```python
from build123d import *

# Parameters (mm, degrees)
F0_W     = 660.4
F0_H     = 571.5
F0_R     = 6.746875
F1_DEPTH = 2.3876
F3_DEPTH = 2.3886
F4_W     = 381
F4_H     = 292.1
F5_DEPTH = 2.3886


with BuildPart() as f1:
    # F0 (on Top) → F1 (new body)
    with BuildSketch(Plane.XY):
        Rectangle(F0_W, F0_H)
        with Locations((-233.3625, -233.3625)):
            Circle(F0_R, mode=Mode.SUBTRACT)
        with Locations((-252.96602, -198.4248)):
            Circle(F0_R, mode=Mode.SUBTRACT)
        with Locations((233.3625, -233.3625)):
            Circle(F0_R, mode=Mode.SUBTRACT)
        with Locations((252.96602, -198.4248)):
            Circle(F0_R, mode=Mode.SUBTRACT)
        with Locations((-233.3625, 233.3625)):
            Circle(F0_R, mode=Mode.SUBTRACT)
        with Locations((0, 239.7252)):
            Circle(F0_R, mode=Mode.SUBTRACT)
        with Locations((233.3625, 233.3625)):
            Circle(F0_R, mode=Mode.SUBTRACT)
    extrude(amount=-F1_DEPTH)

    # F2 (on Top) → F3 (cut, through all)
    with BuildSketch(Plane.XY):
        Polygon((22.225, 285.75), (-22.225, 285.75), (0, 263.525), align=None)
        Polygon((-22.225, -285.75), (22.225, -285.75), (0, -263.525), align=None)
    extrude(amount=-F3_DEPTH, mode=Mode.SUBTRACT)

    # F4 (on Top) → F5 (cut, through all)
    with BuildSketch(Plane.XY):
        Rectangle(F4_W, F4_H)
    extrude(amount=-F5_DEPTH, mode=Mode.SUBTRACT)


solid = f1.part
```
Read the model definition and answer for the solid it produces. Units are mm, in the model's axes. A direction names the side the tool comes from. Round coordinates to 2 decimals unless told otherwise and drop trailing zeros. Write each loop counter-clockwise with the first axis right and the second up, starting at its lowest first coordinate (ties: lowest second). Pieces come first, ordered by that corner, then holes. Notation, with made-up numbers: M 38,-13.5 L 69,-13.5 A27 ccw 69,5.5 Z; hole C 63.5,63 d3. An arc over 180 degrees is marked long. One line per item, written item: value.
Q1. Which of the six approach directions +Z, -Z, +X, -X, +Y, -Y give full straight-line access (tool end or side, diameter ignored) to faces 3 (the flat face through (-10.957, -274.482, -1.177)), 4 (the flat face through (-11.268, 274.793, -1.177)), 5 (the cylindrical face through (-240.103, -233.066, -1.177))?
Data:
face 3: +Z, -Z, -Y
face 4: +Z, -Z, +Y
face 5: +Z, -Z
Q2. Find section B-B on x = -176. Write down the section's boundary in (y, z).
Data:
outline: M -285.75,-2.39 L -146.05,-2.39 L -146.05,0 L -285.75,0 Z; M 146.05,-2.39 L 285.75,-2.39 L 285.75,0 L 146.05,0 Z
Q3. A flat-ended cylindrical pin translates along its axis: pin 1 Ø1.2 at (x, z) = (17.5, -1) entering from -Y (3 decimals). Find the tip coordinate at first contact, or state that the pin passes through.
Data:
pin 1: y = -281.625
Q4. Find section C-C on z = -0.45. Count the separate pieces of the cut face and the enclosed holes in it, plus the area to 3 significant figures.
Data:
separate pieces: 1
enclosed holes: 8
area: 264,000 mm2
Q5. For a pull along X with two mould halves and no side action, classify faces 1 (the flat face through (-5, 195, 0)), 2 (the flat face through (10.957, 274.482, -1.177)) as +X half, -X half, draft (parallel to the pull), parting line (faces both ways), or undercut.
Data:
face 1: draft
face 2: undercut
Q6. Find section A-A on y = 24. Write down the section's boundary in (x, z), plus the area to 3 significant figures.
Data:
outline: M -330.2,-2.39 L -190.5,-2.39 L -190.5,0 L -330.2,0 Z; M 190.5,-2.39 L 330.2,-2.39 L 330.2,0 L 190.5,0 Z
area: 667 mm2
Q7. Straight lines are drawn through the part: line 1 (X direction, y = -44, z = -0.5); line 2 (Y direction, x = -79, z = -0.9); line 3 (X direction, y = -204.5, z = -1.95). For each, find the intervals that lie inside material, in ascending order. Write a range as [from, to].
Data:
line 1: [-330.2, -190.5], [190.5, 330.2]
line 2: [-285.75, -146.05], [146.05, 285.75]
line 3: [-330.2, -255.9], [-250.03, 250.03], [255.9, 330.2]
